Part print with two shaded views. Sizes in mm from the minimum x, y, z corner. A direction names the side the tool comes from. Round coordinates to 2 decimals unless told otherwise and drop trailing zeros. Order: outer loops, then holes, each group sorted by start corner. A loop starts at its lowest first (then second) coordinate and runs counter-clockwise, first axis right, second up. Notation, with made-up numbers: M 72.25,-17 L 119.25,-17 A19 cw 119.25,2 Z; hole C 72,41.5 d9. An arc over 180 degrees is marked long. Return JSON: item names as keys, results as strings. Group by question number.
Item 1: Slice it at C-C on x = 24.75. Write the cut outline in (y, z) (3 decimals), then the cut area to 3 significant figures.
Item 2: Slice it at A-A on z = 4.25. Give the number of separate pieces and of enclosed holes in the cut face.
Item 3: Slice it at D-D on y = 7.25. Write the cut outline in (x, z).
Item 4: Pin check, flat tip, straight feed: pin 1 Ø3 at (y, z) = (4, 3) entering from +X. Stop position of the tip, or through.
Item 5: Probe line 1 along Z through (x, y) = (25.4, 14); line 2 along X through (y, z) = (7.5, 6); line 3 along Y through (x, z) = (17.75, 6) (3 decimals). List the from-to ranges inside material, lowest first.
Item 6: Which spindle directions (+Z, -Z, +X, -X, +Y, -Y) get a long thin tool onto all of the face, cutting with end or side? Do the marked faces 4 and 5. Say none if no direction does.
Item 7: Pull direction X, two halves, no side cores. Call the marked faces 1, 2 and 3: pulls with the +X half, pulls with the -X half, needs draft (parallel to the pull), parting line crosses it, or undercut.
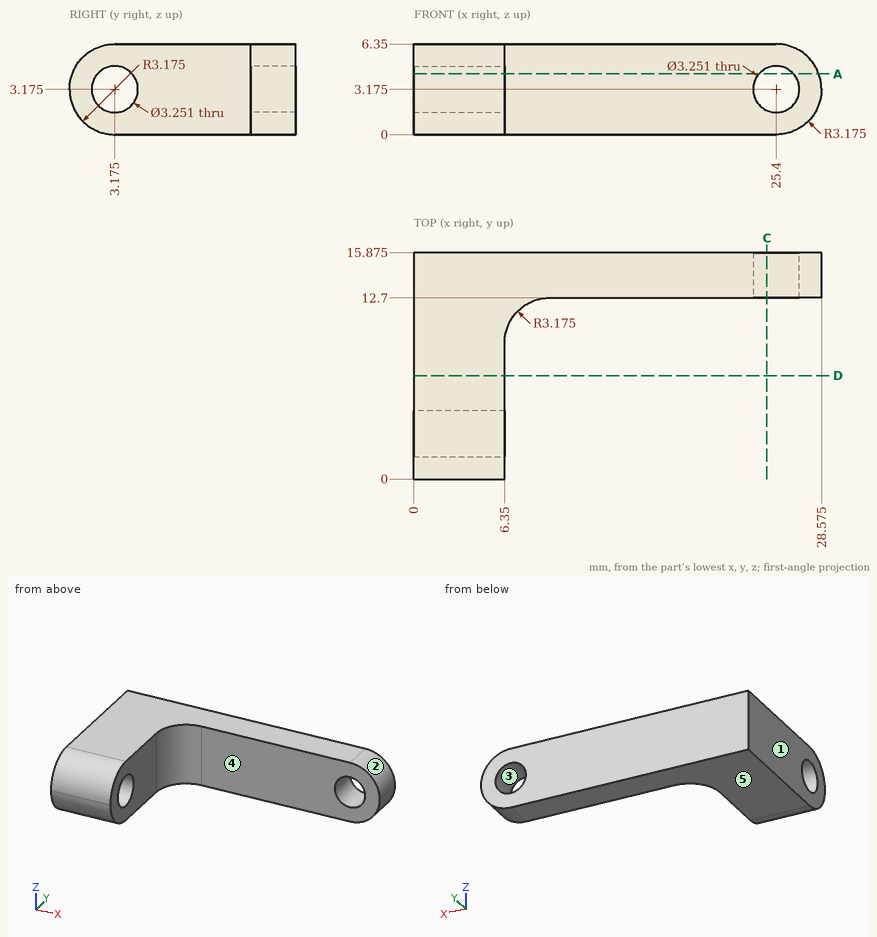
Output values:
{
 "1": {"outline": "M 12.7,0 L 15.875,0 L 15.875,1.685 L 12.7,1.685 Z; M 12.7,4.665 L 15.875,4.665 L 15.875,6.35 L 12.7,6.35 Z", "area": "10.7 mm²"},
 "2": {"separate pieces": "3", "enclosed holes": "0"},
 "3": {"outline": "M 0,0 L 6.35,0 L 6.35,6.35 L 0,6.35 Z"},
 "4": {"pin 1": "x = 6.35"},
 "5": {"line 1": "0 to 1.55, 4.8 to 6.35", "line 2": "0 to 6.35", "line 3": "12.7 to 15.875"},
 "6": {"face 4": "+Z, -Z, +X, -Y", "face 5": "-Z, +X, -X, +Y, -Y"},
 "7": {"face 1": "pulls with the -X half", "face 2": "pulls with the +X half", "face 3": "undercut"}
}
